```python
from build123d import *

# Parameters (mm, degrees)
F0_W        = 25.4
F0_H        = 25.4
F1_DEPTH    = 25.4
F2_SIZE     = 5.08
F3_T1_DEPTH = 25.7610244843
F3_T3_DEPTH = 25.7610244843
F3_T5_DEPTH = 25.7610244843


# Not quite as in the source:
# - a fillet or chamfer that OpenCascade refuses, or shapes differently, is made with other operations: its cross-section is extruded or revolved along the edge and cut away or added


with BuildPart() as f1:
    # F0 (on Front) → F1 (new body)
    with BuildSketch(Plane.XZ):
        with Locations((12.7, 12.7)):
            Rectangle(F0_W, F0_H)
    extrude(amount=F1_DEPTH)

    # F2
    f2_edges = [f1.edges().sort_by_distance(p)[0] for p in [
        (0, -12.7, 25.4),
        (0, -25.4, 12.7),
        (12.7, -25.4, 25.4),
        (0, -12.7, 0),
        (12.7, -25.4, 0),
        (0, 0, 12.7),
        (25.4, -25.4, 12.7),
        (25.4, 0, 12.7),
        (25.4, -12.7, 25.4),
        (25.4, -12.7, 0),
        (12.7, 0, 25.4),
        (12.7, 0, 0),
    ]]
    chamfer(f2_edges, length=F2_SIZE)

    # F3: fillet of radius 5.08 on 24 edges, made by hand

    # F3_s2 → F3_t1 (cut)
    with BuildSketch(Plane.YZ.offset(-0.1805122421)):
        with BuildLine():
            ThreePointArc((-25.4, 18.2157951031), (-25.0133080252, 20.1598269396), (-23.9121024484, 21.8078975516))
            Line((-23.9121024484, 21.8078975516), (-25.4, 20.32))
            Line((-25.4, 20.32), (-25.4, 18.2157951031))
        make_face()
        with BuildLine():
            ThreePointArc((-25.4, 7.1842048969), (-25.0133080252, 5.2401730604), (-23.9121024484, 3.5921024484))
            Line((-23.9121024484, 3.5921024484), (-25.4, 5.08))
            Line((-25.4, 5.08), (-25.4, 7.1842048969))
        make_face()
        with BuildLine():
            ThreePointArc((0, 18.2157951031), (-0.3866919748, 20.1598269396), (-1.4878975516, 21.8078975516))
            Line((-1.4878975516, 21.8078975516), (0, 20.32))
            Line((0, 20.32), (0, 18.2157951031))
        make_face()
        with BuildLine():
            ThreePointArc((0, 7.1842048969), (-0.3866919748, 5.2401730604), (-1.4878975516, 3.5921024484))
            Line((-1.4878975516, 3.5921024484), (0, 5.08))
            Line((0, 5.08), (0, 7.1842048969))
        make_face()
        with BuildLine():
            ThreePointArc((-18.2157951031, 0), (-20.1598269396, 0.3866919748), (-21.8078975516, 1.4878975516))
            Line((-21.8078975516, 1.4878975516), (-20.32, 0))
            Line((-20.32, 0), (-18.2157951031, 0))
        make_face()
        with BuildLine():
            ThreePointArc((-7.1842048969, 0), (-5.2401730604, 0.3866919748), (-3.5921024484, 1.4878975516))
            Line((-3.5921024484, 1.4878975516), (-5.08, 0))
            Line((-5.08, 0), (-7.1842048969, 0))
        make_face()
        with BuildLine():
            ThreePointArc((-18.2157951031, 25.4), (-20.1598269396, 25.0133080252), (-21.8078975516, 23.9121024484))
            Line((-21.8078975516, 23.9121024484), (-20.32, 25.4))
            Line((-20.32, 25.4), (-18.2157951031, 25.4))
        make_face()
        with BuildLine():
            ThreePointArc((-7.1842048969, 25.4), (-5.2401730604, 25.0133080252), (-3.5921024484, 23.9121024484))
            Line((-3.5921024484, 23.9121024484), (-5.08, 25.4))
            Line((-5.08, 25.4), (-7.1842048969, 25.4))
        make_face()
    extrude(amount=F3_T1_DEPTH, mode=Mode.SUBTRACT)

    # F3_s4 → F3_t3 (cut)
    with BuildSketch(Plane.XY.offset(-0.1805122421)):
        with BuildLine():
            ThreePointArc((3.5921024484, -23.9121024484), (5.2401730604, -25.0133080252), (7.1842048969, -25.4))
            Line((7.1842048969, -25.4), (5.08, -25.4))
            Line((5.08, -25.4), (3.5921024484, -23.9121024484))
        make_face()
        with BuildLine():
            ThreePointArc((18.2157951031, -25.4), (20.1598269396, -25.0133080252), (21.8078975516, -23.9121024484))
            Line((21.8078975516, -23.9121024484), (20.32, -25.4))
            Line((20.32, -25.4), (18.2157951031, -25.4))
        make_face()
        with BuildLine():
            ThreePointArc((0, -7.1842048969), (0.3866919748, -5.2401730604), (1.4878975516, -3.5921024484))
            Line((1.4878975516, -3.5921024484), (0, -5.08))
            Line((0, -5.08), (0, -7.1842048969))
        make_face()
        with BuildLine():
            ThreePointArc((0, -18.2157951031), (0.3866919748, -20.1598269396), (1.4878975516, -21.8078975516))
            Line((1.4878975516, -21.8078975516), (0, -20.32))
            Line((0, -20.32), (0, -18.2157951031))
        make_face()
        with BuildLine():
            ThreePointArc((18.2157951031, 0), (20.1598269396, -0.3866919748), (21.8078975516, -1.4878975516))
            Line((21.8078975516, -1.4878975516), (20.32, 0))
            Line((20.32, 0), (18.2157951031, 0))
        make_face()
        with BuildLine():
            ThreePointArc((3.5921024484, -1.4878975516), (5.2401730604, -0.3866919748), (7.1842048969, 0))
            Line((7.1842048969, 0), (5.08, 0))
            Line((5.08, 0), (3.5921024484, -1.4878975516))
        make_face()
        with BuildLine():
            ThreePointArc((23.9121024484, -21.8078975516), (25.0133080252, -20.1598269396), (25.4, -18.2157951031))
            Line((25.4, -18.2157951031), (25.4, -20.32))
            Line((25.4, -20.32), (23.9121024484, -21.8078975516))
        make_face()
        with BuildLine():
            ThreePointArc((23.9121024484, -3.5921024484), (25.0133080252, -5.2401730604), (25.4, -7.1842048969))
            Line((25.4, -7.1842048969), (25.4, -5.08))
            Line((25.4, -5.08), (23.9121024484, -3.5921024484))
        make_face()
    extrude(amount=F3_T3_DEPTH, mode=Mode.SUBTRACT)

    # F3_s6 → F3_t5 (cut)
    with BuildSketch(Plane.XZ.offset(-0.1805122421)):
        with BuildLine():
            ThreePointArc((0, 18.2157951031), (0.3866919748, 20.1598269396), (1.4878975516, 21.8078975516))
            Line((1.4878975516, 21.8078975516), (0, 20.32))
            Line((0, 20.32), (0, 18.2157951031))
        make_face()
        with BuildLine():
            ThreePointArc((0, 7.1842048969), (0.3866919748, 5.2401730604), (1.4878975516, 3.5921024484))
            Line((1.4878975516, 3.5921024484), (0, 5.08))
            Line((0, 5.08), (0, 7.1842048969))
        make_face()
        with BuildLine():
            ThreePointArc((23.9121024484, 21.8078975516), (25.0133080252, 20.1598269396), (25.4, 18.2157951031))
            Line((25.4, 18.2157951031), (25.4, 20.32))
            Line((25.4, 20.32), (23.9121024484, 21.8078975516))
        make_face()
        with BuildLine():
            ThreePointArc((23.9121024484, 3.5921024484), (25.0133080252, 5.2401730604), (25.4, 7.1842048969))
            Line((25.4, 7.1842048969), (25.4, 5.08))
            Line((25.4, 5.08), (23.9121024484, 3.5921024484))
        make_face()
        with BuildLine():
            ThreePointArc((3.5921024484, 1.4878975516), (5.2401730604, 0.3866919748), (7.1842048969, 0))
            Line((7.1842048969, 0), (5.08, 0))
            Line((5.08, 0), (3.5921024484, 1.4878975516))
        make_face()
        with BuildLine():
            ThreePointArc((18.2157951031, 0), (20.1598269396, 0.3866919748), (21.8078975516, 1.4878975516))
            Line((21.8078975516, 1.4878975516), (20.32, 0))
            Line((20.32, 0), (18.2157951031, 0))
        make_face()
        with BuildLine():
            ThreePointArc((18.2157951031, 25.4), (20.1598269396, 25.0133080252), (21.8078975516, 23.9121024484))
            Line((21.8078975516, 23.9121024484), (20.32, 25.4))
            Line((20.32, 25.4), (18.2157951031, 25.4))
        make_face()
        with BuildLine():
            ThreePointArc((3.5921024484, 23.9121024484), (5.2401730604, 25.0133080252), (7.1842048969, 25.4))
            Line((7.1842048969, 25.4), (5.08, 25.4))
            Line((5.08, 25.4), (3.5921024484, 23.9121024484))
        make_face()
    extrude(amount=F3_T5_DEPTH, mode=Mode.SUBTRACT)


solid = f1.part
```
The model under review builds one solid part; all positions refer to its coordinate system, in mm. Round coordinates to 2 decimals unless told otherwise and drop trailing zeros. Order: outer loops, then holes, each group sorted by start corner. A loop starts at its lowest first (then second) coordinate and runs counter-clockwise, first axis right, second up. Notation, with made-up numbers: M 54,23 L 105,23 A25 cw 105,52 Z; hole C 86.25,-12 d10. An arc over 180 degrees is marked long. Use a Markdown table: item, result.
1) Insertion check: pin 1 (1.5 mm diameter, centred on x = 4, z = 7, fed in from +Y); pin 2 (8 mm diameter, centred on x = 4, y = -16.5, fed in from +Z); pin 3 (1 mm diameter, centred on x = 13.5, z = 4.5, fed in from +Y). Each pin has a flat end and moves straight along its axis. Give the tip position at first contact, or say it passes through.
Report:
| item | result |
|---|---|
| pin 1 | y = -0.62 |
| pin 2 | z = 25.4 |
| pin 3 | y = -0.49 |
2) Consider section D-D (x = 11.5). Write out the cut boundary in (y, z), then the cut area to 3 significant figures.
Report:
| item | result |
|---|---|
| outline | M -25.4,7.18 A5.08 ccw -23.91,3.59 L -21.81,1.49 A5.08 ccw -18.22,0 L -7.18,0 A5.08 ccw -3.59,1.49 L -1.49,3.59 A5.08 ccw 0,7.18 L 0,18.22 A5.08 ccw -1.49,21.81 L -3.59,23.91 A5.08 ccw -7.18,25.4 L -18.22,25.4 A5.08 ccw -21.81,23.91 L -23.91,21.81 A5.08 ccw -25.4,18.22 Z |
| area | 589 mm^2 |
3) Consider section C-C (z = 17). Write out the cut boundary in (x, y).
Report:
| item | result |
|---|---|
| outline | M 0,-18.22 A5.08 ccw 1.49,-21.81 L 3.59,-23.91 A5.08 ccw 7.18,-25.4 L 18.22,-25.4 A5.08 ccw 21.81,-23.91 L 23.91,-21.81 A5.08 ccw 25.4,-18.22 L 25.4,-7.18 A5.08 ccw 23.91,-3.59 L 21.81,-1.49 A5.08 ccw 18.22,0 L 7.18,0 A5.08 ccw 3.59,-1.49 L 1.49,-3.59 A5.08 ccw 0,-7.18 Z |
4) Wall thickness on line 1 along Z through (x, y) = (14.25, -5.75); line 2 along X through (y, z) = (-5.25, 9.75); line 3 along Y through (x, z) = (6.25, 14.5): over which ranges is each line inside the solid? List them lowest first. Write a range as [from, to].
Report:
| item | result |
|---|---|
| line 1 | [0.21, 25.19] |
| line 2 | [0.38, 25.02] |
| line 3 | [-25.31, -0.09] |
5) Consider section B-B (y = -2.5). Write out the cut boundary in (x, z).
Report:
| item | result |
|---|---|
| outline | M 2.58,5.08 L 5.08,2.58 L 20.32,2.58 L 22.82,5.08 L 22.82,20.32 L 20.32,22.82 L 5.08,22.82 L 2.58,20.32 Z |
6) Consider section A-A (x = 2.75). Write out the cut boundary in (y, z).
Report:
| item | result |
|---|---|
| outline | M -23.07,5.08 L -20.32,2.33 L -5.08,2.33 L -2.33,5.08 L -2.33,20.32 L -5.08,23.07 L -20.32,23.07 L -23.07,20.32 Z |
